from build123d import *

# Parameters (mm, degrees)
SKETCH1_R             = 6
BOSS_EXTRUDE1_DEPTH   = 28
BOSS_EXTRUDE1_2_DEPTH = 28
SKETCH2_R             = 56
BOSS_EXTRUDE3_DEPTH   = 30
SKETCH3_R             = 15
CUT_EXTRUDE1_DEPTH    = 29


with BuildPart() as part:
    # Sketch1 → Boss-Extrude1 (new body)
    with BuildSketch(Plane(origin=(0, 0, 0), x_dir=(1, 0, 0), z_dir=(0, 1, 0))):
        with Locations(Location((43.301270189, -75, 0), (0, 0, 270))):
            Circle(SKETCH1_R)
    extrude(amount=BOSS_EXTRUDE1_DEPTH)



with BuildPart() as body_2:
    # Sketch1 → Boss-Extrude1 2 (new body)
    with BuildSketch(Plane(origin=(0, 0, 0), x_dir=(1, 0, 0), z_dir=(0, 1, 0))):
        with BuildLine():
            ThreePointArc((0, -70), (9.54447402, -94.489495355), (25.980762114, -115))
            ThreePointArc((25.980762114, -115), (-25.980762114, -115), (0, -70))
        make_face()
    extrude(amount=BOSS_EXTRUDE1_2_DEPTH)


with BuildPart() as part_1:
    add(part.part)

    add(body_2.part)  # Boss-Extrude3 merges body 2
    # Sketch2 → Boss-Extrude3 (add)
    with BuildSketch(Plane(origin=(0, 0, 0), x_dir=(1, 0, 0), z_dir=(0, 1, 0))):
        with Locations(Location((0, -100, 0), (0, 0, 270))):
            Circle(SKETCH2_R)
    extrude(amount=-BOSS_EXTRUDE3_DEPTH)

    # Sketch3 → Cut-Extrude1 (cut)
    with BuildSketch(Plane.XZ.offset(30)):
        with Locations(Location((0, 100, 0), (0, 0, 270))):
            Circle(SKETCH3_R)
    extrude(amount=-CUT_EXTRUDE1_DEPTH, mode=Mode.SUBTRACT)


solid = part_1.part
Could you check a few things on this model? Use its own coordinates, in mm. A direction names the side the tool comes from. Give positions to 0.01 mm unless a question says otherwise; leave off trailing zeros. Order: outer loops, then holes, each group sorted by start corner. A loop starts at its lowest first (then second) coordinate and runs counter-clockwise, first axis right, second up. Notation, with made-up numbers: (-23, 8) - (28, 8) arc R29 ccw to (28, 45) - close; hole circle Ø8 at (3, -24.75). An arc over 180 degrees is marked (long way). One line per question, with ' | ' between items. Start each with the question number.
Item 1: I want a section at A-A on z = 128. Write out the boundary of the cut face in (x, y).
Item 2: For faces 4 (the flat face through (-8, 28, 106)), 5 (the cylindrical face through (-25.5, 13.8, 115.8)), 6 (the flat face through (0, -1, 100)), 7 (the cylindrical face through (9.36, 13.8, 94.17)), which set-ups out of +Z, -Z, +X, -X, +Y, -Y let a thin tool reach every point of the face, with its end or its side?
Item 3: I want a section at D-D on z = 88. Write out the boundary of the cut face in (x, y), then the cut area to 3 significant figures.
Item 4: I want a section at C-C on x = -11.5. Write out the boundary of the cut face in (y, z), then the cut area to 3 significant figures.
Item 5: Thinking about a two-plate mould opening in X: for faces 1 (the flat face through (-12, -30, 112)), 2 (the cylindrical face through (-21.45, -14.79, 151.73)), 3 (the cylindrical face through (43.565, 13.804, 69.006)), which applies, pulls with the +X half, pulls with the -X half, needs draft (parallel to the pull), parting line crosses it, or undercut?
Item 6: I'm going to push flat-ended pins straight in: pin 1 Ø1.5 at (y, z) = (15, 114) entering from +X; pin 2 Ø1 at (y, z) = (16.5, 78) entering from -X; pin 3 Ø6 at (y, z) = (10.5, 83.5) entering from +X. Where does each tip first touch, or does it pass through?
Item 7: I want a section at B-B on y = -3. Write out the boundary of the cut face in (x, z), then the cut area to 3 significant figures.
Item 8: I need wall thicknesses on probe 1 along X at (y, z) = (-8, 100); probe 2 along Y at (x, z) = (-5, 140); probe 3 along Z at (x, y) = (-9, -18.5). Which ranges of each line are inside material? Lowest first, please. Write a range as [from, to].
Verdict:
1) outline: (-48.5, -30) - (48.5, -30) - (48.5, 0) - (10.77, 0) - (10.77, 28) - (-10.77, 28) - (-10.77, 0) - (-48.5, 0) - close
2) face 4: +Z, -Z, +X, -X, +Y | face 5: +Y | face 6: -Y | face 7: -Z, +Y
3) outline: (-54.7, -30) - (-9, -30) - (-9, -1) - (9, -1) - (9, -30) - (54.7, -30) - (54.7, 0) - (6.15, 0) - (6.15, 28) - (-27.5, 28) - (-27.5, 0) - (-54.7, 0) - close | area: 3,700 mm^2
4) outline: (-30, 45.19) - (0, 45.19) - (0, 72.29) - (28, 72.29) - (28, 127.71) - (0, 127.71) - (0, 154.81) - (-30, 154.81) - (-30, 109.63) - (-1, 109.63) - (-1, 90.37) - (-30, 90.37) - close | area: 4,280 mm^2
5) face 1: needs draft | face 2: parting line crosses it | face 3: undercut
6) pin 1: x = 25.71 | pin 2: x = -20.92 | pin 3: x = 45.7
7) outline: circle Ø112 at (0, 100); hole circle Ø30 at (0, 100) | area: 9,150 mm^2
8) probe 1: [-56, -15], [15, 56] | probe 2: [-30, 0] | probe 3: [44.73, 88], [112, 155.27]
